Read the model definition and answer for the solid it produces. Units are mm, in the model's axes. A direction names the side the tool comes from. Coordinates: 2 decimals unless noted, no trailing zeros. Write each loop counter-clockwise with the first axis right and the second up, starting at its lowest first coordinate (ties: lowest second). Pieces come first, ordered by that corner, then holes. Notation, with made-up numbers: (5.5, 88) -> (59.5, 88) arc R26 ccw to (59.5, 102) -> close; hole circle Ø10 at (-39.5, 10). An arc over 180 degrees is marked (long way). One line per item, written item: value. Start each with the question number.
1. Given P1, Ø3, axis at y = 35, z = 6, coming from the -X side; P2, Ø0.6, axis at y = 9, z = 9, coming from the -X side; P3, Ø5.5, axis at x = 10, z = 6.5, coming from the +Y side; P4, Ø18, axis at x = 40, y = 26, coming from the -Z side, each flat-ended and moving along its own axis, determine where each tip first touches the part or whether it passes through.
2. For faces 4 (the flat face through (12, 8, 4)), 5 (the flat face through (54, 21, 7)), 6 (the cylindrical face through (33.06, 26.91, 6.41)), determine the directions among +Z, -Z, +X, -X, +Y, -Y from which every point of the face is accessible in a straight line to the end or side of a thin tool.
3. Consider line 1 along X through (y, z) = (2.75, 6.5); line 2 along X through (y, z) = (4, 4.75); line 3 along Z through (x, y) = (70, 2.5). Determine where each line is inside the solid, lowest interval first.
4. Find section C-C, the plane z = 11. Write down the section's boundary in (x, y).
5. Find section B-B, the plane x = 40. Write down the section's boundary in (y, z), and give its area (3 significant figures).
6. For a pull along X with two mould halves and no side action, classify faces 1 (the cylindrical face through (25, 12, 6)), 2 (the flat face through (72, 8, 4)), 3 (the cylindrical face through (72.4, 3.95, 5.97)) as pulls with the +X half, pulls with the -X half, needs draft (parallel to the pull), parting line crosses it, or undercut.
7. Find section D-D, the plane y = 6.5. Write down the section's boundary in (x, z).
8. Find section A-A, the plane z = 6.5. State how many separate pieces and enclosed holes the cut face has, and give its area (3 significant figures).
Autodesk Inventor part; units mm, degrees
ref_plane "YZ Plane" through (0, 0, 0) normal (1, 0, 0) x (0, 1, 0)
ref_plane "XZ Plane" through (0, 0, 0) normal (0, 1, 0) x (-1, 0, 0)
ref_plane "XY Plane" through (0, 0, 0) normal (0, 0, 1) x (1, 0, 0)
sketch "Sketch1" plane through (0, 0, 0) normal (0, 0, 1) x (1, 0, 0)
  line L0 (0, 0) -> (80, 0)
  line L1 (80, 0) -> (80, 40)
  line L2 (80, 40) -> (0, 40)
  line L3 (0, 40) -> (0, 0)
  dimension "d0" = 80
  dimension "d1" = 40
extrude "Extrusion1" add sketch "Sketch1" along normal blind 13
sketch "Sketch2" plane through (0, 0, 13) normal (0, 0, 1) x (1, 0, 0)
  line L0 (80, 0) -> (0, 0)
  line L1 (80, 40) -> (80, 0)
  point P0 (40, 26)
  dimension "d4" = 26
  dimension "d5" = 40
hole "Hole1" at (40, 26, 13) direction (0, 0, -1) diameter 14 depth 13 tip angle 118
sketch "Sketch3" plane through (0, 0, 13) normal (0, 0, 1) x (1, 0, 0)
  circle A0 centre (40, 26) radius 7
  line L0 (0, 0) -> (0, 40)
  line L1 (80, 0) -> (0, 0)
  line L2 (80, 40) -> (80, 0)
  line L3 (0, 40) -> (80, 40)
  arc A1 (54, 26) -> (26, 26) centre (40, 26) ccw
  line L4 (54, 26) -> (54, 10)
  line L5 (26, 26) -> (26, 10)
  line L6 (0, 10) -> (26, 10)
  line L7 (54, 10) -> (80, 10)
  dimension "d14" = 10
  dimension "d15" = 10
  dimension "d16" = 26
extrude "Extrusion2" cut sketch "Sketch3" against normal blind 13 contours L0 L3 A1 L5 L6 | L7 L4 A1 L3 L2
sketch "Sketch6" plane through (54, 10, 13) normal (0, 1, 0) x (1, 0, 0)
  line L0 (0, 13) -> (26, 13)
  line L1 (0, 0) -> (0, 13)
  line L2 (26, 0) -> (0, 0)
  line L3 (26, 13) -> (26, 0)
  line L4 (-54, 13) -> (-28, 13)
  line L5 (-54, 0) -> (-54, 13)
  line L6 (-28, 0) -> (-54, 0)
  line L7 (-28, 0) -> (-28, 13)
  line L8 (-34, 13) -> (-34, 0)
  line L9 (6, 13) -> (6, 0)
  point P0 (-54, 13)
  dimension "d36" = 40
  dimension "d37" = 6
extrude "Extrusion4" cut sketch "Sketch6" against normal blind 2 contours L0 L3 L2 L9 | L4 L8 L6 L5
sketch "Sketch7" plane through (54, 8, 13) normal (0, 1, 0) x (1, 0, 0)
  line L0 (-54, 13) -> (-34, 13)
  line L1 (-54, 0) -> (-54, 13)
  line L2 (6, 13) -> (6, 0)
  line L3 (26, 0) -> (6, 0)
  line L4 (26, 13) -> (26, 0)
  line L5 (6, 13) -> (26, 13)
  point P0 (-44, 6.5)
  point P1 (16, 6.5)
  dimension "d40" = 60
  dimension "d41" = 6.5
  dimension "d42" = 10
hole "Hole3" at (10, 8, 6.5) at (70, 8, 6.5) direction (0, -1, 0) diameter 4.917 depth 8 tip angle 118
chamfer "Chamfer1" distance 0.5 angle 45 4 edges at (10, 8, 4.0415) (70, 8, 4.0415) (10, 0, 4.0415) (70, 0, 4.0415)
fillet "Fillet2" radius 5 2 edges at (26, 10, 6.5) (54, 10, 6.5)
properties part number "MANCAL DA BETONEIRA(26)" material "Carbon Steel"
Answer block:
1. P1: stops at x = 28.18
1. P2: stops at x = 20
1. P3: stops at y = 7.79
1. P4: stops at z = 0
2. face 4: +Z, -Z, -X, +Y
2. face 5: +Z, -Z, +X, +Y
2. face 6: +Z, -Z
3. line 1: x = 0 to 7.54, 12.46 to 67.54, 72.46 to 80
3. line 2: x = 0 to 8.27, 11.73 to 68.27, 71.73 to 80
3. line 3: z = 0 to 4.04, 8.96 to 13
4. outline: (0, 0) -> (80, 0) -> (80, 8) -> (60, 8) -> (60, 10) -> (59, 10) arc R5 cw to (54, 15) -> (54, 26) arc R14 ccw to (26, 26) -> (26, 15) arc R5 cw to (21, 10) -> (20, 10) -> (20, 8) -> (0, 8) -> close; hole circle Ø14 at (40, 26)
5. outline: (0, 0) -> (19, 0) -> (19, 13) -> (0, 13) -> close; (33, 0) -> (40, 0) -> (40, 13) -> (33, 13) -> close
5. area: 338 mm2
6. face 1: pulls with the -X half
6. face 2: needs draft
6. face 3: undercut
7. outline: (0, 0) -> (80, 0) -> (80, 13) -> (0, 13) -> close; hole circle Ø4.92 at (10, 6.5); hole circle Ø4.92 at (70, 6.5)
8. separate pieces: 3
8. enclosed holes: 1
8. area: 1,250 mm2
